For this review, take the finished solid that the model builds, in its own axes (mm). Give positions to 0.01 mm unless a question says otherwise; leave off trailing zeros. Write each loop counter-clockwise with the first axis right and the second up, starting at its lowest first coordinate (ties: lowest second). Pieces come first, ordered by that corner, then holes. Notation, with made-up numbers: (-0.75, 37) -> (39.25, 37) arc R17 ccw to (39.25, 41) -> close; hole circle Ø8 at (8, -37.75). An arc over 180 degrees is marked (long way). Write item = value, one per line.
Autodesk Inventor part; units mm, degrees
ref_plane "YZ Plane" through (0, 0, 0) normal (1, 0, 0) x (0, 1, 0)
ref_plane "XZ Plane" through (0, 0, 0) normal (0, 1, 0) x (-1, 0, 0)
ref_plane "XY Plane" through (0, 0, 0) normal (0, 0, 1) x (1, 0, 0)
sketch "Sketch1" plane through (0, 0, 0) normal (0, 1, 0) x (-1, 0, 0)
  line L0 (-57.6, 57.6) -> (57.6, 57.6)
  line L1 (57.6, 57.6) -> (57.6, -57.6)
  line L2 (57.6, -57.6) -> (-57.6, -57.6)
  line L3 (-57.6, -57.6) -> (-57.6, 57.6)
  line L4 (-57.6, 57.6) -> (57.6, -57.6) construction
  line L5 (57.6, 57.6) -> (-57.6, -57.6) construction
  circle A0 centre (52.4, 52.4) radius 1.5
  circle A1 centre (52.4, -52.4) radius 1.5
  arc A2 (56.1, 27.5507) -> (27.5507, 56.1) centre (0, 0) ccw
  arc A3 (27.5507, -56.1) -> (56.1, -27.5507) centre (0, 0) ccw
  arc A4 (-56.1, -27.5507) -> (-27.5507, -56.1) centre (0, 0) ccw
  arc A5 (-27.5507, 56.1) -> (-56.1, 27.5507) centre (0, 0) ccw
  line L6 (27.5507, 56.1) -> (-27.5507, 56.1)
  line L7 (-56.1, 27.5507) -> (-56.1, -27.5507)
  line L8 (-27.5507, -56.1) -> (27.5507, -56.1)
  line L9 (56.1, -27.5507) -> (56.1, 27.5507)
  arc A6 (57.6, 52.4) -> (52.4, 57.6) centre (52.4, 52.4) ccw
  line L10 (47.7863, 57.6) -> (44.1942, 44.1942)
  line L11 (44.1942, 44.1942) -> (57.6, 47.7863)
  line L12 (-58, 58) -> (58, 58) construction
  line L13 (58, 58) -> (58, -58) construction
  line L14 (58, -58) -> (-58, -58) construction
  line L15 (-58, -58) -> (-58, 58) construction
  line L16 (-58, 58) -> (58, -58) construction
  line L17 (58, 58) -> (-58, -58) construction
  circle A7 centre (52.4, 52.4) radius 3
  point P0 (0, 56.1)
  dimension "d1" = 3
  dimension "d2" = 104.8
  dimension "d4" = 62.5
  dimension "d9" = 30
  dimension "d80" = 116
  dimension "d81" = 0.4
  dimension "d82" = 1.5
  dimension "d88" = 6
extrude "Extrusion3" add sketch "Sketch1" along normal blind 2.775 contours L0 L10 L11 L1 L2 L3 | L0 A6 L1 L11 L10 | L0 L1 A6 | A0 | A1 | A7
extrude "Extrusion5" cut sketch "Sketch1" along normal up to next contours L0 L1 A6
sketch "Sketch4" plane through (0, 2.775, 0) normal (0, 1, 0) x (1, 0, 0)
  line L0 (-56.1, -27.5507) -> (-56.1, 27.5507)
  arc A0 (-27.5507, 56.1) -> (-56.1, 27.5507) centre (0, 0) ccw
  line L1 (-27.5507, 56.1) -> (27.5507, 56.1)
  arc A1 (56.1, 27.5507) -> (27.5507, 56.1) centre (0, 0) ccw
  line L2 (56.1, 27.5507) -> (56.1, -27.5507)
  arc A2 (27.5507, -56.1) -> (56.1, -27.5507) centre (0, 0) ccw
  line L3 (27.5507, -56.1) -> (-27.5507, -56.1)
  arc A3 (-56.1, -27.5507) -> (-27.5507, -56.1) centre (0, 0) ccw
  line L4 (-57.6, 57.6) -> (-57.6, -52.4)
  arc A4 (-57.6, -52.4) -> (-52.4, -57.6) centre (-52.4, -52.4) ccw
  line L5 (-52.4, -57.6) -> (57.6, -57.6)
  line L6 (57.6, -57.6) -> (57.6, 57.6)
  line L7 (57.6, 57.6) -> (-57.6, 57.6)
  circle A5 centre (0, 0) radius 28
  circle A6 centre (0, 0) radius 29.5
  line L8 (52.4, 52.4) -> (-52.4, -52.4) construction
  line L9 (-21.3832, -20.3226) -> (-44.7213, -43.6607)
  line L10 (-43.6607, -44.7213) -> (-20.3226, -21.3832)
  arc A7 (-52.4, 56.1) -> (-56.1, 52.4) centre (-52.4, 52.4) ccw
  line L11 (-56.1, 52.4) -> (-56.1, -52.4)
  arc A8 (-56.1, -52.4) -> (-52.4, -56.1) centre (-52.4, -52.4) ccw
  line L12 (-52.4, -56.1) -> (52.4, -56.1)
  arc A9 (52.4, -56.1) -> (56.1, -52.4) centre (52.4, -52.4) ccw
  line L13 (56.1, -52.4) -> (56.1, 52.4)
  arc A10 (56.1, 52.4) -> (52.4, 56.1) centre (52.4, 52.4) ccw
  line L14 (52.4, 56.1) -> (-52.4, 56.1)
  arc A11 (-52.4, 55.2) -> (-55.2, 52.4) centre (-52.4, 52.4) ccw
  line L15 (-55.2, 52.4) -> (-55.2, -52.4)
  arc A12 (-55.2, -52.4) -> (-52.4, -55.2) centre (-52.4, -52.4) ccw
  line L16 (-52.4, -55.2) -> (52.4, -55.2)
  arc A13 (52.4, -55.2) -> (55.2, -52.4) centre (52.4, -52.4) ccw
  line L17 (55.2, -52.4) -> (55.2, 52.4)
  arc A14 (55.2, 52.4) -> (52.4, 55.2) centre (52.4, 52.4) ccw
  line L18 (52.4, 55.2) -> (-52.4, 55.2)
  arc A15 (-56.1, -27.5507) -> (-27.5507, -56.1) centre (0, 0) ccw
  arc A16 (-55.2, -29.3123) -> (-29.3123, -55.2) centre (0, 0) ccw
  circle A17 centre (0, 0) radius 44.1942 construction
  line L19 (0, 44.1942) -> (44.1942, 44.1942) construction
  circle A18 centre (0, 0) radius 44.9442
  circle A19 centre (0, 0) radius 43.4442
  point P0 (0, 0)
  dimension "d36" = 56
  dimension "d37" = 1.5
  dimension "d38" = 1.5
  dimension "d48" = 0.9
  dimension "d69" = 1.5
  dimension "d70" = 0.75
extrude "Extrusion12" add sketch "Sketch4" against normal blind 2.775 contours A18 L10 A19 L9 | L9 A19 L10 A18 | A6
extrude "Extrusion13" add sketch "Sketch4" against normal blind 2.775 contours L9 A18 L10 A3 | L9 A19 L10 A18 | L9 A6 L10 A19 picked at (-30.6576, -31.4825) picked at (-23.7298, -24.5548)
extrude "Extrusion15" cut sketch "Sketch1" along normal up to next contours A0
extrude "Extrusion16" cut sketch "Sketch1" along normal blind 1.3875 contours A7
pattern_circular "Circular Pattern8" count 4 over 360 about axis through (0, 2.775, 0) along (0, -1, 0) of "Extrusion15", "Extrusion16", "Extrusion13", "Extrusion5"
equation "\"d1\" = holeSize"
equation "\"d2\" = dHoles"
equation "\"d4\" = 0.5 * fanDia"
equation "\"d82\" = d39"
equation "\"d22\" = thickness"
equation "\"d36\" = fanCenter"
equation "\"d37\" = d39"
equation "\"d38\" = d39"
equation "\"d69\" = d39"
equation "\"d70\" = 0.5 * d39"
equation "\"d62\" = thickness"
equation "\"d64\" = thickness"
equation "\"d89\" = 0.5 * thickness"
equation "\"holeSize\" = 3"
equation "\"thickness\" = 2.775"
properties part number "intake2"
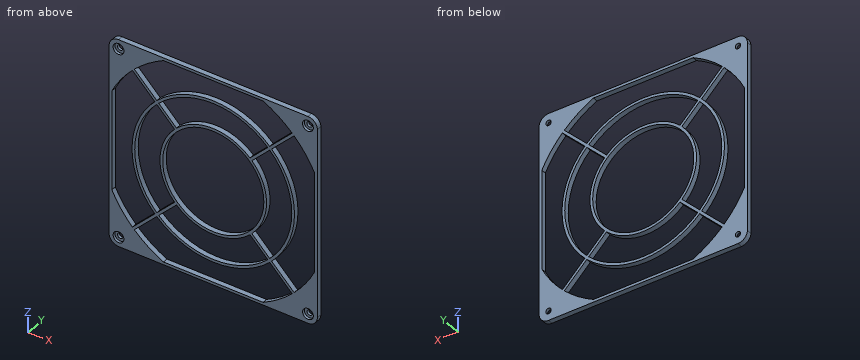
(1) Take a section at C-C (x = 23). Count the separate pieces of the cut face and the enclosed holes in it, plus the area to 3 significant figures.
Answers below:
separate_pieces = 8
enclosed_holes = 0
area = 43.7 mm^2
(2) For pin 1 (5 mm diameter, centred on x = 52.4, z = -52.4, fed in from -Y), flat-tipped, find the tip position at first contact; note if it passes through.
Answers below:
pin_1 = 1.39
(3) Take a section at B-B (z = 0). Write out the cut boundary in (x, y) (3 decimals), plus the area to 3 significant figures.
Answers below:
outline = (-57.6, 0) -> (-56.1, 0) -> (-56.1, 2.775) -> (-57.6, 2.775) -> close; (-44.944, 0) -> (-43.444, 0) -> (-43.444, 2.775) -> (-44.944, 2.775) -> close; (-29.5, 0) -> (-28, 0) -> (-28, 2.775) -> (-29.5, 2.775) -> close; (28, 0) -> (29.5, 0) -> (29.5, 2.775) -> (28, 2.775) -> close; (43.444, 0) -> (44.944, 0) -> (44.944, 2.775) -> (43.444, 2.775) -> close; (56.1, 0) -> (57.6, 0) -> (57.6, 2.775) -> (56.1, 2.775) -> close
area = 25.0 mm^2
(4) To check wall thickness, follow probe 1 along X at (y, z) = (2.65, 1); probe 2 along X at (y, z) = (0.5, 37.5); probe 3 along Z at (x, y) = (36.5, 0.9). State the ranges of each line that lie inside material, in increasing order.
Answers below:
probe_1 = -57.6 to -56.1, -44.93 to -43.43, -29.48 to -27.98, 27.98 to 29.48, 43.43 to 44.93, 56.1 to 57.6
probe_2 = -57.6 to -50, -38.56 to -36.44, -24.77 to -21.94, 21.94 to 24.77, 36.44 to 38.56, 50 to 57.6
probe_3 = -57.6 to -50.73, -37.56 to -35.44, -26.22 to -23.56, 23.56 to 26.22, 35.44 to 37.56, 50.73 to 57.6
(5) Take a section at A-A (x = 0). Write out the cut boundary in (y, z) (3 decimals).
Answers below:
outline = (0, -57.6) -> (2.775, -57.6) -> (2.775, -56.1) -> (0, -56.1) -> close; (0, -44.944) -> (2.775, -44.944) -> (2.775, -43.444) -> (0, -43.444) -> close; (0, -29.5) -> (2.775, -29.5) -> (2.775, -28) -> (0, -28) -> close; (0, 28) -> (2.775, 28) -> (2.775, 29.5) -> (0, 29.5) -> close; (0, 43.444) -> (2.775, 43.444) -> (2.775, 44.944) -> (0, 44.944) -> close; (0, 56.1) -> (2.775, 56.1) -> (2.775, 57.6) -> (0, 57.6) -> close
